Check sheet for the drawn part. Datum: minimum x, y, z corner. Units: mm. Give positions to 0.01 mm unless a question says otherwise; leave off trailing zeros. Write each loop counter-clockwise with the first axis right and the second up, starting at its lowest first coordinate (ties: lowest second). Pieces come first, ordered by that corner, then holes. Notation, with made-up numbers: (-21, -33) -> (-9, -33) arc R33 cw to (-9, 5) -> close; hole circle Ø3 at (47.25, -2.5). An arc over 180 degrees is marked (long way). Answer as CSV lines item,"result". Start each with the question number.
1) Sectioned sample at A-A on z = 37.5. Record the cut outline in (x, y), and give its area (3 significant figures).
2) Sectioned sample at B-B on x = 13. Record the cut outline in (y, z), and give its area (3 significant figures).
3) Sectioned sample at C-C on y = 4.1. Record the cut outline in (x, z), and give its area (3 significant figures).
4) Material ranges on L1, parallel to Z at x = 34, y = 2.15; L2, parallel to X at y = 0.5, z = 33; L3, parallel to Z at x = 61.5, y = 0.3, recorded low to high.
5) Sectioned sample at D-D on z = 18. Record the cut outline in (x, y), and give its area (3 significant figures).
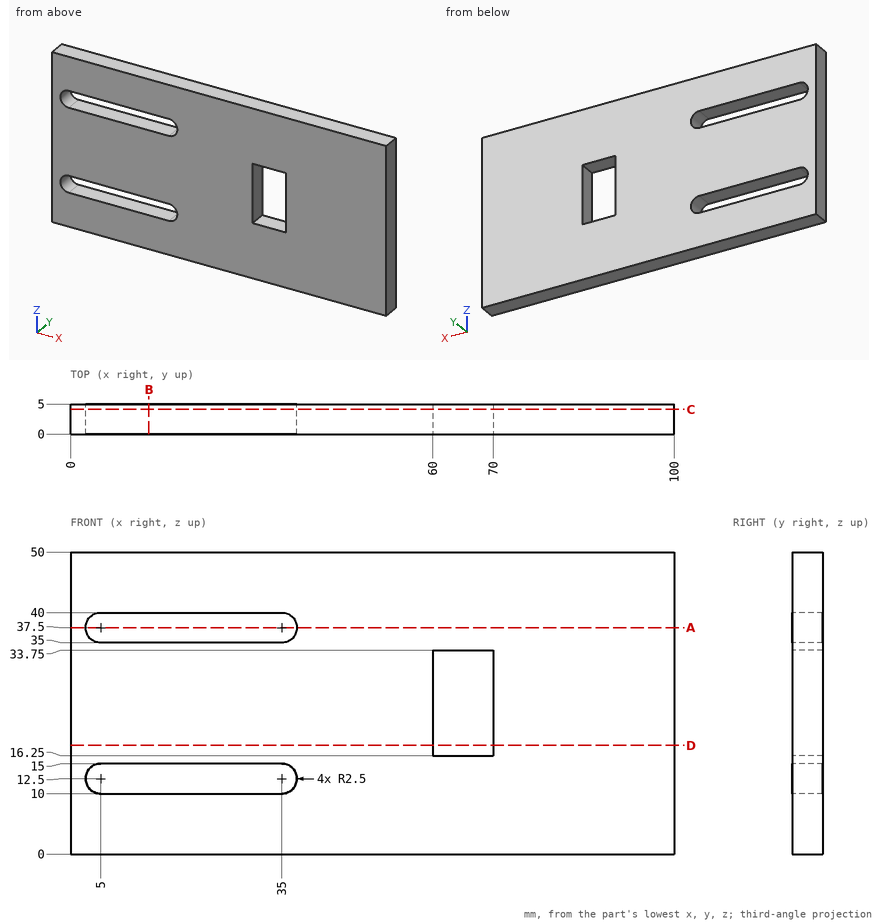
Ans:
1,outline,"(0, 0) -> (2.5, 0) -> (2.5, 5) -> (0, 5) -> close; (37.5, 0) -> (100, 0) -> (100, 5) -> (37.5, 5) -> close"
1,area,"325 mm²"
2,outline,"(0, 0) -> (5, 0) -> (5, 10) -> (0, 10) -> close; (0, 15) -> (5, 15) -> (5, 35) -> (0, 35) -> close; (0, 40) -> (5, 40) -> (5, 50) -> (0, 50) -> close"
2,area,"200 mm²"
3,outline,"(0, 0) -> (100, 0) -> (100, 50) -> (0, 50) -> close; hole (5, 10) -> (35, 10) arc R2.5 ccw to (35, 15) -> (5, 15) arc R2.5 ccw to start; hole (5, 35) -> (35, 35) arc R2.5 ccw to (35, 40) -> (5, 40) arc R2.5 ccw to start; hole (60, 16.25) -> (70, 16.25) -> (70, 33.75) -> (60, 33.75) -> close"
3,area,"4,490 mm²"
4,L1,"z = 0 to 10, 15 to 35, 40 to 50"
4,L2,"x = 0 to 60, 70 to 100"
4,L3,"z = 0 to 16.25, 33.75 to 50"
5,outline,"(0, 0) -> (60, 0) -> (60, 5) -> (0, 5) -> close; (70, 0) -> (100, 0) -> (100, 5) -> (70, 5) -> close"
5,area,"450 mm²"
